Can you work these out from the model? Positions are in its coordinate system, mm. Face numbers are marked on the shaded views. Round coordinates to 2 decimals unless told otherwise and drop trailing zeros. Loops run counter-clockwise (first coordinate to the right, second up) from the corner with the lowest first, then second, coordinate; pieces in that order, holes last. Notation, with made-up numbers: (31, 75) - (79, 75) arc R23 ccw to (79, 107) - close; hole circle Ø10 at (28.5, 86.5). An arc over 180 degrees is marked (long way). Answer as CSV lines item,"result".
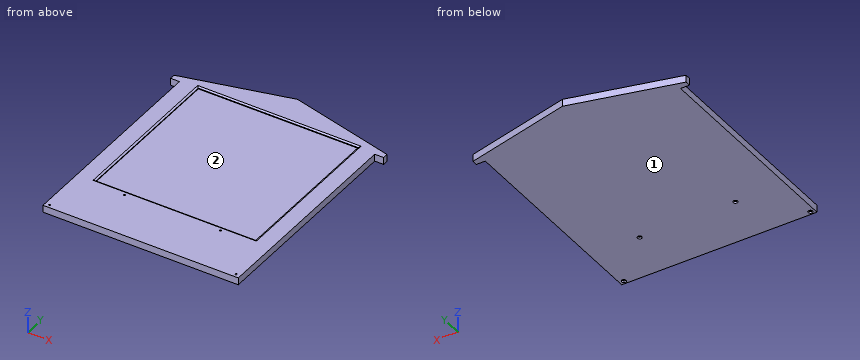
```python
from build123d import *

# Parameters (mm, degrees)
SKETCH_1_W          = 110
SKETCH_1_H          = 4
EXTRUDE_1_DEPTH     = 120
SKETCH_2_W          = 120
SKETCH_2_H          = 4
EXTRUDE_2_DEPTH     = 18
CUT_EXTRUDE_1_DEPTH = 5
SKETCH_4_W          = 90
SKETCH_4_H          = 90
CUT_EXTRUDE_2_DEPTH = 1
SKETCH_6_R          = 0.5
CUT_EXTRUDE_3_DEPTH = 5
SKETCH_7_R          = 1.25
CUT_EXTRUDE_4_DEPTH = 1
CHAMFER_1_SIZE      = 1
CHAMFER_1_SIZE2     = 0.577350269


with BuildPart() as part:
    # 草图1 → 凸台-拉伸1 (new body)
    with BuildSketch(Plane(origin=(0, 0, 0), x_dir=(1, 0, 0), z_dir=(0, 1, 0))):
        Rectangle(SKETCH_1_W, SKETCH_1_H)
    extrude(amount=EXTRUDE_1_DEPTH)

    # 草图2 → 凸台-拉伸2 (add)
    with BuildSketch(Plane(origin=(0, 120, 0), x_dir=(1, 0, 0), z_dir=(0, 1, 0))):
        Rectangle(SKETCH_2_W, SKETCH_2_H)
    extrude(amount=EXTRUDE_2_DEPTH)

    # 草图3 → 切除-拉伸1 (cut, through all)
    with BuildSketch(Plane.XY.offset(2)):
        Polygon((-60, 138), (0, 138), (-60, 123), align=None)
    cut_extrude_1 = extrude(amount=-CUT_EXTRUDE_1_DEPTH, mode=Mode.SUBTRACT)

    # 镜向1: 切除-拉伸1 across plane
    add(cut_extrude_1.mirror(Plane(origin=(0, 0, 0), x_dir=(0, 0, 1), z_dir=(1, 0, 0))), mode=Mode.SUBTRACT)

    # 草图4 → 切除-拉伸2 (cut)
    with BuildSketch(Plane.XY.offset(2)):
        with Locations((0, 76)):
            Rectangle(SKETCH_4_W, SKETCH_4_H)
    extrude(amount=-CUT_EXTRUDE_2_DEPTH, mode=Mode.SUBTRACT)

    # 草图6 → 切除-拉伸3 (cut, through all)
    with BuildSketch(Plane(origin=(0, 0, -2), x_dir=(-1, 0, 0), z_dir=(0, 0, -1))):
        with Locations((-52.5, 2)):
            Circle(SKETCH_6_R)
        with Locations((-27, 28)):
            Circle(SKETCH_6_R)
        with Locations((27, 28)):
            Circle(SKETCH_6_R)
        with Locations((52.5, 2)):
            Circle(SKETCH_6_R)
    extrude(amount=-CUT_EXTRUDE_3_DEPTH, mode=Mode.SUBTRACT)

    # 草图7 → 切除-拉伸4 (cut)
    with BuildSketch(Plane(origin=(0, 0, -2), x_dir=(-1, 0, 0), z_dir=(0, 0, -1))):
        with Locations((-52.5, 2)):
            Circle(SKETCH_7_R)
        with Locations((-27, 28)):
            Circle(SKETCH_7_R)
        with Locations((27, 28)):
            Circle(SKETCH_7_R)
        with Locations((52.5, 2)):
            Circle(SKETCH_7_R)
    extrude(amount=-CUT_EXTRUDE_4_DEPTH, mode=Mode.SUBTRACT)

    # 倒角1
    chamfer_1_edges = [part.edges().sort_by_distance(p)[0] for p in [
        (-45, 76, 2),
        (0, 31, 2),
        (45, 76, 2),
        (0, 121, 2),
    ]]
    chamfer_1_side = [part.faces().sort_by_distance(p)[0] for p in [
        (57.5, 121.828770078, 2),
    ]]
    chamfer(chamfer_1_edges, length=CHAMFER_1_SIZE, length2=CHAMFER_1_SIZE2, reference=chamfer_1_side[0])


solid = part.part
```
Q1. Imagine slicing it at A-A (z = -0.2). Write out the boundary of the cut face in (x, y), then the cut area to 3 significant figures.
Checks:
outline,"(-60, 120) - (-55, 120) - (-55, 0) - (55, 0) - (55, 120) - (60, 120) - (60, 123) - (0, 138) - (-60, 123) - close; hole circle Ø1 at (-52.5, 2); hole circle Ø1 at (-27, 28); hole circle Ø1 at (27, 28); hole circle Ø1 at (52.5, 2)"
area,"14,500 mm²"
Q2. We'd pull the mould along Y, two halves only. Please class the marked faces 1 and 2: pulls with the +Y half, pulls with the -Y half, needs draft (parallel to the pull), parting line crosses it, or undercut.
Checks:
face 1,"needs draft"
face 2,"undercut"
Q3. I'm going to push flat-ended pins straight in: pin 1 Ø2 at (x, y) = (-27, 28) entering from -Z; pin 2 Ø1.2 at (y, z) = (36.5, 0) entering from -X; pin 3 Ø0.8 at (x, y) = (-52.5, 2) entering from -Z; pin 4 Ø4 at (x, y) = (-28.5, 46.5) entering from +Z. Where does each tip first touch, or does it pass through?
Checks:
pin 1,"z = -1"
pin 2,"x = -55"
pin 3,"through"
pin 4,"z = 1"
Q4. Imagine slicing it at C-C (y = 94). Write out the boundary of the cut face in (x, z), then the cut area to 3 significant figures.
Checks:
outline,"(-55, -2) - (55, -2) - (55, 2) - (46, 2) - (45, 1.42) - (45, 1) - (-45, 1) - (-45, 1.42) - (-46, 2) - (-55, 2) - close"
area,"349 mm²"
Q5. Imagine slicing it at B-B (x = 21). Write out the boundary of the cut face in (y, z), then the cut area to 3 significant figures.
Checks:
outline,"(0, -2) - (132.75, -2) - (132.75, 2) - (122, 2) - (121, 1.42) - (121, 1) - (31, 1) - (31, 1.42) - (30, 2) - (0, 2) - close"
area,"440 mm²"
Q6. Imagine slicing it at D-D (y = 17). Write out the boundary of the cut face in (x, z).
Checks:
outline,"(-55, -2) - (55, -2) - (55, 2) - (-55, 2) - close"
Q7. If I drill on line 1 along Z through (x, y) = (16, 58.5); line 2 along X through (y, z) = (71.5, -0.2); line 3 along Y through (x, z) = (-27, -1.5), over which ranges is the centre line in solid material (lowest first)? Write a range as [from, to].
Checks:
line 1,"[-2, 1]"
line 2,"[-55, 55]"
line 3,"[0, 26.75], [29.25, 131.25]"
